from build123d import *

# Parameters (mm, degrees)
F0_W     = 4.2024515569
F0_H     = 12.3226391152
F1_DEPTH = 25


with BuildPart() as f1:
    # F0 (on Front) → F1 (new body)
    with BuildSketch(Plane.XZ):
        with Locations((22.6418208331, -0.4750718363)):
            Rectangle(F0_W, F0_H)
    extrude(amount=F1_DEPTH)


with BuildPart() as f1b:
    # F0 (on Front) → F1, piece 2 (new body)
    with BuildSketch(Plane.XZ):
        Polygon((52.4395957523, 24.4672579743), (43.5876576167, 33.9897979507), (24.0114504894, 15.7921978513), (27.5258704588, 12.0115337595), (24.0114504894, 8.7446083143), (27.4481885135, 5.3967726417), (30.8740026641, 8.5813321185), (32.9489489509, 6.3491928217), align=None)
    extrude(amount=F1_DEPTH)


solid = f1b.part
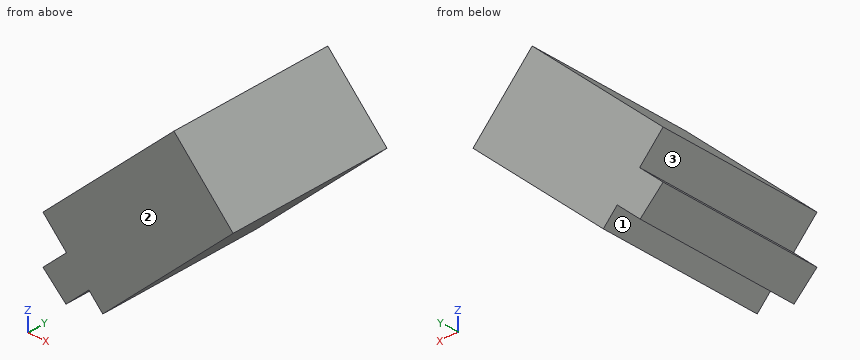
Design review of the part built by this model. Coordinates are the model's own, in mm. Face numbers are marked on the shaded views. Round coordinates to 2 decimals unless told otherwise and drop trailing zeros. Loops run counter-clockwise (first coordinate to the right, second up) from the corner with the lowest first, then second, coordinate; pieces in that order, holes last. Notation, with made-up numbers: (84, -27) - (110, -27) arc R10 cw to (110, -8) - close; hole circle Ø11 at (69.5, 43.5). An arc over 180 degrees is marked (long way). One line per item, written item: value. Start each with the question number.
1) Consider section C-C on z = 7.75. Give the boundary of the cut face in (x, y).
2) Draft analysis for pull direction Z (two halves, no side actions). For the marked faces 1, 2 and 3, state which applies: +Z half, -Z half, draft (parallel to the pull), parting line (faces both ways), or undercut.
3) To check wall thickness, follow L1, parallel to Z at x = 27, y = -16.25; L2, parallel to Z at x = 25.75, y = -20; L3, parallel to X at y = -22.5, z = 15.5. State the ranges of each line that lie inside material, in increasing order. Write a range as from..to.
4) Insertion check: pin 1 Ø4 at (x, y) = (44, -14.5) entering from -Z; pin 2 Ø1.5 at (y, z) = (-22, 30) entering from +X; pin 3 Ø8 at (y, z) = (-15, 16.5) entering from -X; pin 4 Ø10 at (y, z) = (-10, 26.5) entering from -X. Each pin has a flat end and moves straight along its axis. Give the tip position at first contact, or say it passes through.
5) Consider section B-B on x = 26.5. Give the boundary of the cut face in (y, z), then the cut area to 3 significant figures.
6) Consider section D-D on z = 31. Give the boundary of the cut face in (x, y), then the cut area to 3 significant figures.
7) Consider section A-A on y = -4. Give the boundary of the cut face in (x, z).
Reported:
1. outline: (25.03, -25) - (29.98, -25) - (29.98, 0) - (25.03, 0) - close; (31.65, -25) - (34.46, -25) - (34.46, 0) - (31.65, 0) - close
2. face 1: -Z half
2. face 2: draft
2. face 3: undercut
3. L1: z = 5.83..11.52, 12.58..18.57
3. L2: z = 7.05..10.36, 13.92..17.41
3. L3: x = 24.28..42.79
4. pin 1: stops at z = 14.76
4. pin 2: stops at x = 47.99
4. pin 3: stops at x = 24.01
4. pin 4: stops at x = 30.15
5. outline: (-25, 6.32) - (0, 6.32) - (0, 11.06) - (-25, 11.06) - close; (-25, 13.12) - (0, 13.12) - (0, 18.11) - (-25, 18.11) - close
5. area: 243 mm^2
6. outline: (40.37, -25) - (46.37, -25) - (46.37, 0) - (40.37, 0) - close
6. area: 150 mm^2
7. outline: (24.01, 8.74) - (27.45, 5.4) - (30.87, 8.58) - (32.95, 6.35) - (52.44, 24.47) - (43.59, 33.99) - (24.01, 15.79) - (27.53, 12.01) - close
